from build123d import *

# Parameters (mm, degrees)
F2_R           = 30
F2_R_2         = 10
F5_DEPTH       = 27.5
F6_R           = 2
F7_D           = 4.2
F7_DEPTH       = 22
F7_CBORE_D     = 9.75
F7_CBORE_DEPTH = 5
F7_TIP         = 1.2618073
F8_D           = 4.2
F8_DEPTH       = 22
F8_CBORE_D     = 9.75
F8_CBORE_DEPTH = 5
F8_TIP         = 1.2618073


with BuildPart() as f5:
    # F2 (on Right) → F5 (new body, symmetric)
    with BuildSketch(Plane.YZ):
        Circle(F2_R)
        Circle(F2_R_2, mode=Mode.SUBTRACT)
    extrude(amount=F5_DEPTH, both=True)

    # F6
    f6_edges = [f5.edges().sort_by_distance(p)[0] for p in [
        (27.5, -30, 0),
        (-27.5, -30, 0),
    ]]
    fillet(f6_edges, radius=F6_R)

    # F7
    with Locations(Plane.XY.offset(30)):
        with Locations((-12.5, 0), (12.5, 0)):
            CounterBoreHole(F7_D / 2, F7_CBORE_D / 2, F7_CBORE_DEPTH, depth=F7_DEPTH)
            with Locations((0, 0, -(F7_DEPTH + F7_TIP / 2))):  # 118° drill point
                Cone(0, F7_D / 2, F7_TIP, mode=Mode.SUBTRACT)

    # F8
    with Locations(Plane(origin=(0, 0, -30), x_dir=(1, 0, 0), z_dir=(0, 0, -1))):
        with Locations((0, 0)):
            CounterBoreHole(F8_D / 2, F8_CBORE_D / 2, F8_CBORE_DEPTH, depth=F8_DEPTH)
            with Locations((0, 0, -(F8_DEPTH + F8_TIP / 2))):  # 118° drill point
                Cone(0, F8_D / 2, F8_TIP, mode=Mode.SUBTRACT)


solid = f5.part
Check sheet for the modelled part. Datum: model origin and axes. Units: mm. A direction names the side the tool comes from. Round coordinates to 2 decimals unless told otherwise and drop trailing zeros. Loops run counter-clockwise (first coordinate to the right, second up) from the corner with the lowest first, then second, coordinate; pieces in that order, holes last.
1. Sectioned sample at B-B on x = -12.5. Record the boundary of the cut face in (y, z) (3 decimals).
2. Set-up check for faces 1 (the cylindrical face through (0.357, -6.503, -29.287)), 2 (the flat face through (15, -1, 25)), 3 (the cylindrical face through (-4.87, -0.21, -27.54)): record each of +Z, -Z, +X, -X, +Y, -Y from which the full face is reachable in a straight line by a thin tool's end or side.
3. Gauge pin test, flat ends, axial feed: pin 1 Ø1.5 at (x, y) = (6.5, -8.5) entering from +Z; pin 2 Ø3 at (x, y) = (6.5, -7) entering from +Z; pin 3 Ø3 at (x, y) = (-9, -5) entering from -Z. Record the tip position at first contact, or that the pin passes through.
4. Sectioned sample at A-A on x = 20. Record the boundary of the cut face in (y, z), and give its area (3 significant figures).
5. Sectioned sample at C-C on z = 21. Give the number of separate pieces and of enclosed holes in the cut face, and give its area (3 significant figures).
6. Mould release check, pull along X, two halves, no side actions. Record for faces 4 (the flat face through (27.5, 0, -12)), 5 (the cylindrical face through (14.6, 0.09, 17.28)), 6 (the flat face through (-27.5, 0, -12)): released by +X, released by -X, zero draft, split by the parting line, or undercut.
7. Scan lines: probe 1 along X at (y, z) = (0, 14); probe 2 along Z at (x, y) = (-8.5, -1.5); probe 3 along Y at (x, z) = (0, -17). Record each from-to range of solid material in increasing order.
8. Sectioned sample at D-D on x = -4. Record the boundary of the cut face in (y, z), and give its area (3 significant figures).
Recorded:
1. outline: (-4.875, 25) - (-4.875, 29.601) arc R30 ccw (long way) to (4.875, 29.601) - (4.875, 25) - (2.1, 25) - (2.1, 9.777) arc R10 cw (long way) to (-2.1, 9.777) - (-2.1, 25) - close
2. face 1: +X, -X
2. face 2: +Z
2. face 3: -Z
3. pin 1: stops at z = 28.98
3. pin 2: stops at z = 29.49
3. pin 3: stops at z = -29.8
4. outline: circle Ø60 at (0, 0); hole circle Ø20 at (0, 0)
4. area: 2,510 mm2
5. separate pieces: 1
5. enclosed holes: 2
5. area: 2,320 mm2
6. face 4: released by +X
6. face 5: undercut
6. face 6: released by -X
7. probe 1: x = -27.5 to -14.6, -10.4 to 10.4, 14.6 to 27.5
7. probe 2: z = -29.96 to -9.89, 9.89 to 25
7. probe 3: y = -24.72 to -2.1, 2.1 to 24.72
8. outline: (-2.79, -29.87) - (-2.79, -25) - (2.79, -25) - (2.79, -29.87) arc R30 ccw (long way) to start; hole circle Ø20 at (0, 0)
8. area: 2,490 mm2
